Geometry: see drawing. Coordinates: mm, zero at the bounding-box minimum. A direction names the side the tool comes from. Round coordinates to 2 decimals unless told otherwise and drop trailing zeros. Loops run counter-clockwise (first coordinate to the right, second up) from the corner with the lowest first, then second, coordinate; pieces in that order, holes last.
(1) Material intervals for probe 1 along Z at (x, y) = (0.85, 0.25); probe 2 along Y at (x, z) = (1.3, 7.25); probe 3 along Z at (x, y) = (0.5, 1.05), sorted ascending.
(2) Section C-C, the plane z = 10. Return the cut outline in (x, y), plus the area to 3 significant figures.
(3) Set-up query: the marked faces 1, 2 and 3. Return all of +Z, -Z, +X, -X, +Y, -Y with unobstructed straight access to the full face (end or side cutting, diameter ignored); none if empty.
(4) Section A-A, the plane x = 1.27. Return the cut outline in (y, z).
(5) First-contact query: pin 1 Ø0.5 at (x, y) = (1, 1.5) entering from +Z; pin 2 Ø1.3 at (x, y) = (2, 2) entering from +Z. Flat tips, straight axial feed; report the tip coordinate or a pass-through.
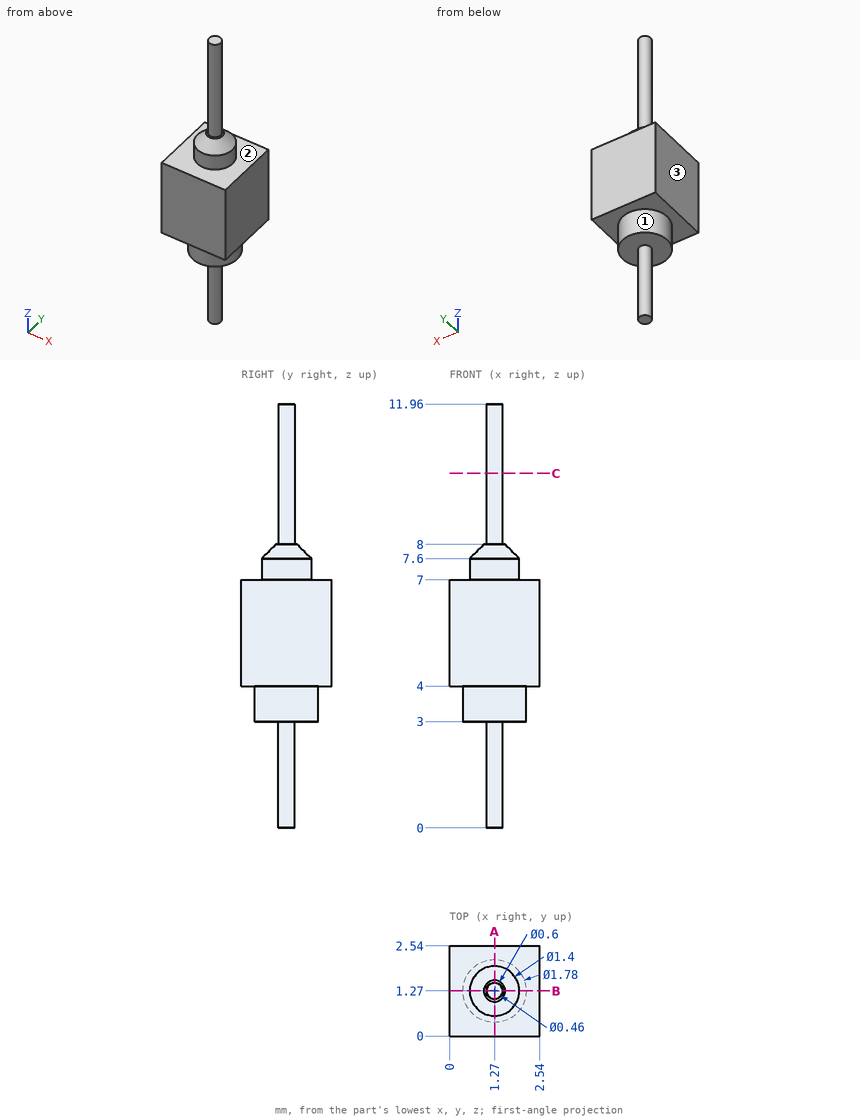
Output values:
1. probe 1: z = 4 to 7
1. probe 2: y = 0.57 to 1.97
1. probe 3: z = 3 to 7
2. outline: circle Ø0.46 at (1.27, 1.27)
2. area: 0.166 mm2
3. face 1: -Z
3. face 2: +Z
3. face 3: +Z, -Z, -X, +Y, -Y
4. outline: (0, 4) - (0.38, 4) - (0.38, 3) - (1.04, 3) - (1.04, 0) - (1.5, 0) - (1.5, 3) - (2.16, 3) - (2.16, 4) - (2.54, 4) - (2.54, 7) - (1.97, 7) - (1.97, 7.6) - (1.57, 8) - (1.5, 8) - (1.5, 11.96) - (1.04, 11.96) - (1.04, 8) - (0.97, 8) - (0.57, 7.6) - (0.57, 7) - (0, 7) - close
5. pin 1: stops at z = 11.96
5. pin 2: stops at z = 7.92
